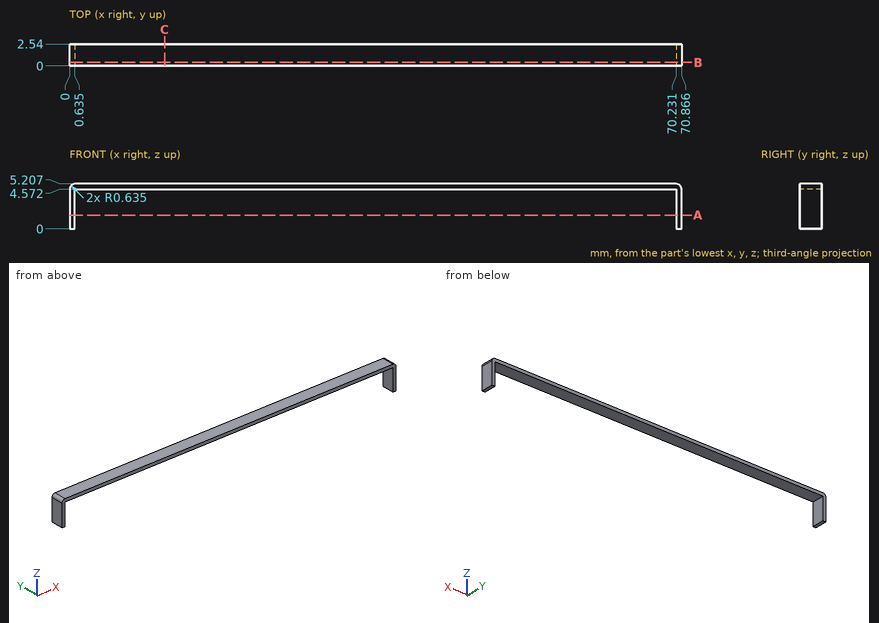
Input: dimensioned drawing with shaded views. Units: mm. Origin: part minimum x, y, z. Give positions to 0.01 mm unless a question says otherwise; leave off trailing zeros. Write each loop counter-clockwise with the first axis right and the second up, starting at its lowest first coordinate (ties: lowest second). Pieces come first, ordered by that corner, then holes. Notation, with made-up numbers: (63, -2) -> (68, -2) arc R19 cw to (68, 23) -> close; hole circle Ø5 at (85.25, 38). An arc over 180 degrees is marked (long way). Answer as a JSON object with one key per item and string values.
1. Ray query, probe 1 along X at (y, z) = (0.8, 1.95) (3 decimals); probe 2 along Z at (x, y) = (30, 1.1); probe 3 along X at (y, z) = (1.7, 4.75). Return the intervals inside material, ascending. Write a range as from..to.
Ans:
{"probe 1": "x = 0..0.635, 70.231..70.866", "probe 2": "z = 4.57..5.21", "probe 3": "x = 0.03..70.84"}
2. Cut plane C-C on x = 11. Output: boundary loops of the cut face in (y, z), and give its area (3 significant figures).
Ans:
{"outline": "(0, 4.57) -> (2.54, 4.57) -> (2.54, 5.21) -> (0, 5.21) -> close", "area": "1.61 mm^2"}
3. Cut plane B-B on y = 0.4. Output: boundary loops of the cut face in (x, z) (3 decimals), and give its area (3 significant figures).
Ans:
{"outline": "(0, 0) -> (0.635, 0) -> (0.635, 4.572) -> (70.231, 4.572) -> (70.231, 0) -> (70.866, 0) -> (70.866, 4.572) arc R0.635 ccw to (70.231, 5.207) -> (0.635, 5.207) arc R0.635 ccw to (0, 4.572) -> close", "area": "50.6 mm^2"}
4. Cut plane A-A on z = 1.6. Output: boundary loops of the cut face in (x, y) (3 decimals).
Ans:
{"outline": "(0, 0) -> (0.635, 0) -> (0.635, 2.54) -> (0, 2.54) -> close; (70.231, 0) -> (70.866, 0) -> (70.866, 2.54) -> (70.231, 2.54) -> close"}
